```python
from build123d import *

# Parameters (mm, degrees)
SKETCH_1_W          = 106
SKETCH_1_H          = 45
EXTRUDE_1_DEPTH     = 200
SKETCH_2_W          = 86
SKETCH_2_H          = 180
CUT_EXTRUDE_1_DEPTH = 35
SKETCH_3_R          = 7.5
CUT_EXTRUDE_2_DEPTH = 210.842798304
SKETCH_4_W          = 24.030592061
SKETCH_4_H          = 7.207958271
CUT_EXTRUDE_4_DEPTH = 35
SKETCH_5_W          = 106
SKETCH_5_H          = 200
EXTRUDE_2_DEPTH     = 5


with BuildPart() as part:
    # 草圖1 → 填料-伸長1 (new body)
    with BuildSketch(Plane(origin=(0, 0, 0), x_dir=(1, 0, 0), z_dir=(0, 1, 0))):
        Rectangle(SKETCH_1_W, SKETCH_1_H)
    extrude(amount=EXTRUDE_1_DEPTH)

    # 草圖2 → 除料-伸長1 (cut)
    with BuildSketch(Plane.XY.offset(22.5)):
        with Locations((0, 100)):
            Rectangle(SKETCH_2_W, SKETCH_2_H)
    extrude(amount=-CUT_EXTRUDE_1_DEPTH, mode=Mode.SUBTRACT)

    # 草圖3 → 除料-伸長2 (cut, through all)
    with BuildSketch(Plane.XY.offset(-12.5)):
        with Locations((-26.696570332, 150.301958836)):
            Circle(SKETCH_3_R)
        with Locations((-1.696570332, 150.301958836)):
            Circle(SKETCH_3_R)
        with Locations((23.303429668, 150.301958836)):
            Circle(SKETCH_3_R)
    extrude(amount=-CUT_EXTRUDE_2_DEPTH, mode=Mode.SUBTRACT)

    # 草圖4 → 除料-伸長4 (cut)
    with BuildSketch(Plane.XZ):
        with Locations((-20.984703969, 10.896020865)):
            Rectangle(SKETCH_4_W, SKETCH_4_H)
    extrude(amount=-CUT_EXTRUDE_4_DEPTH, mode=Mode.SUBTRACT)

    # 草圖5 → 填料-伸長2 (add)
    with BuildSketch(Plane.XY.offset(22.5)):
        with Locations((0, 100)):
            Rectangle(SKETCH_5_W, SKETCH_5_H)
    extrude(amount=EXTRUDE_2_DEPTH)


solid = part.part
```
Geometry: final body of the model. Coordinates: model frame, mm. A direction names the side the tool comes from. Coordinates: 2 decimals unless noted, no trailing zeros. Loops run counter-clockwise (first coordinate to the right, second up) from the corner with the lowest first, then second, coordinate; pieces in that order, holes last. Notation, with made-up numbers: (2.25, 0) -> (25.25, 0) arc R19 cw to (25.25, 32) -> close; hole circle Ø8 at (64.5, 70.25). An arc over 180 degrees is marked (long way). Use a Markdown table: item, result. Add a question column.
(1) Section query B-B, the plane y = 104. Return loops of the section in (x, z), plus the area to 3 significant figures.
(2) Section query D-D, the plane z = -16. Return loops of the section in (x, y), plus the area to 3 significant figures.
(3) Mould query, pull axis X, two halves, no side actions, for faces 1 (the flat face through (-33, 5, 11)), 2 (the flat face through (-1, 101, 27.5)), 3 (the flat face through (53, 99, 2)), 4 (the flat face through (-53, 99, 2)). Classes: pulls with the +X half, pulls with the -X half, needs draft (parallel to the pull), parting line crosses it, or undercut.
(4) Section query A-A, the plane x = -38. Return loops of the section in (y, z).
(5) Line query: line 1 along Z through (x, y) = (5, 170); line 2 along X through (y, z) = (16, 10); line 3 along Y through (x, z) = (10, -11.5). Output: solid intervals per line, ascending.
(6) Access query for faces 5 (the flat face through (-21, 5, 14.5)), 6 (the cylindrical face through (-9.19, 150.63, -17.43)), 7 (the flat face through (-1, 0, 2)), 8 (the flat face through (-43, 99, 5)). Directions: +Z, -Z, +X, -X, +Y, -Y. A direction counts if a zero-diameter tool reaches every point of the face in a straight line with its end or side. Return the directions, or none.
(7) Section query C-C, the plane y = 155. Return loops of the section in (x, z), plus the area to 3 significant figures.
(8) Pin query (flat end, axial travel): pin 1 Ø13.5 at (x, y) = (23.3, 150.3) entering from -Z; pin 2 Ø5 at (x, z) = (-23, 11.5) entering from -Y. Return the tip coordinate at first contact, or that it passes through.
Answer:
| question | item | result |
|---|---|---|
| 1 | outline | (-53, -22.5) -> (53, -22.5) -> (53, 27.5) -> (-53, 27.5) -> close; hole (-43, -12.5) -> (43, -12.5) -> (43, 22.5) -> (-43, 22.5) -> close |
| 1 | area | 2,290 mm^2 |
| 2 | outline | (-53, 0) -> (53, 0) -> (53, 200) -> (-53, 200) -> close; hole circle Ø15 at (-26.7, 150.3); hole circle Ø15 at (-1.7, 150.3); hole circle Ø15 at (23.3, 150.3) |
| 2 | area | 20,700 mm^2 |
| 3 | face 1 | undercut |
| 3 | face 2 | needs draft |
| 3 | face 3 | pulls with the +X half |
| 3 | face 4 | pulls with the -X half |
| 4 | outline | (0, -22.5) -> (200, -22.5) -> (200, 27.5) -> (0, 27.5) -> close; hole (10, -12.5) -> (190, -12.5) -> (190, 22.5) -> (10, 22.5) -> close |
| 5 | line 1 | z = -22.5 to -12.5, 22.5 to 27.5 |
| 5 | line 2 | x = -53 to -43, 43 to 53 |
| 5 | line 3 | y = 0 to 10, 190 to 200 |
| 6 | face 5 | -Y |
| 6 | face 6 | -Z |
| 6 | face 7 | +Z, -Z, +X, -X, -Y |
| 6 | face 8 | none |
| 7 | outline | (-53, -22.5) -> (-32.54, -22.5) -> (-32.54, -12.5) -> (-43, -12.5) -> (-43, 22.5) -> (43, 22.5) -> (43, -12.5) -> (29.15, -12.5) -> (29.15, -22.5) -> (53, -22.5) -> (53, 27.5) -> (-53, 27.5) -> close; (-20.85, -22.5) -> (-7.54, -22.5) -> (-7.54, -12.5) -> (-20.85, -12.5) -> close; (4.15, -22.5) -> (17.46, -22.5) -> (17.46, -12.5) -> (4.15, -12.5) -> close |
| 7 | area | 1,940 mm^2 |
| 8 | pin 1 | stops at z = 22.5 |
| 8 | pin 2 | stops at y = 190 |
